```python
from build123d import *

# Parameters (mm, degrees)
SKETCH_R         = 44
SKETCH_R_2       = 30
PAD_DEPTH        = 5
SKETCH001_R      = 44
SKETCH001_R_2    = 41
PAD001_DEPTH     = 65
SKETCH002_R      = 44
SKETCH002_R_2    = 34
PAD002_DEPTH     = 5
HOLE_D           = 3.6
HOLE_DEPTH       = 5
HOLE_CBORE_D     = 6.2
HOLE_CBORE_DEPTH = 3
CHAMFER_SIZE     = 6.9
FILLET_R         = 1
CHAMFER001_SIZE  = 1
CHAMFER002_SIZE  = 3.8
FILLET001_R      = 3
CHAMFER003_SIZE  = 0.2


with BuildPart() as part:
    # Sketch → Pad (new body)
    with BuildSketch(Plane.XY):
        Circle(SKETCH_R)
        Circle(SKETCH_R_2, mode=Mode.SUBTRACT)
    extrude(amount=PAD_DEPTH)

    # Sketch001 (on DatumPlane) → Pad001 (join)
    with BuildSketch(Plane.XY.offset(5)):
        Circle(SKETCH001_R)
        Circle(SKETCH001_R_2, mode=Mode.SUBTRACT)
    extrude(amount=PAD001_DEPTH)

    # Sketch002 (on DatumPlane) → Pad002 (join)
    with BuildSketch(Plane.XY.offset(70)):
        Circle(SKETCH002_R)
        Circle(SKETCH002_R_2, mode=Mode.SUBTRACT)
    extrude(amount=PAD002_DEPTH)

    # Hole
    with Locations(Plane.XY.offset(5)):
        with Locations((-36.6, 0), (18.3, 31.69653), (18.3, -31.69653)):
            CounterBoreHole(HOLE_D / 2, HOLE_CBORE_D / 2, HOLE_CBORE_DEPTH, depth=HOLE_DEPTH)

    # Chamfer
    chamfer_edges = [part.edges().sort_by_distance(p)[0] for p in [
        (-41, 0, 70),
    ]]
    chamfer(chamfer_edges, length=CHAMFER_SIZE)

    # Fillet
    fillet_edges = [part.edges().sort_by_distance(p)[0] for p in [
        (-34, 0, 75),
        (-44, 0, 75),
    ]]
    fillet(fillet_edges, radius=FILLET_R)

    # Chamfer001
    chamfer001_edges = [part.edges().sort_by_distance(p)[0] for p in [
        (-41, 0, 5),
    ]]
    chamfer(chamfer001_edges, length=CHAMFER001_SIZE)

    # Chamfer002
    chamfer002_edges = [part.edges().sort_by_distance(p)[0] for p in [
        (-44, 0, 0),
    ]]
    chamfer(chamfer002_edges, length=CHAMFER002_SIZE)

    # Fillet001
    fillet001_edges = [part.edges().sort_by_distance(p)[0] for p in [
        (-30, 0, 5),
    ]]
    fillet(fillet001_edges, radius=FILLET001_R)

    # Chamfer003
    chamfer003_edges = [part.edges().sort_by_distance(p)[0] for p in [
        (-30, 0, 0),
    ]]
    chamfer(chamfer003_edges, length=CHAMFER003_SIZE)


solid = part.part
```
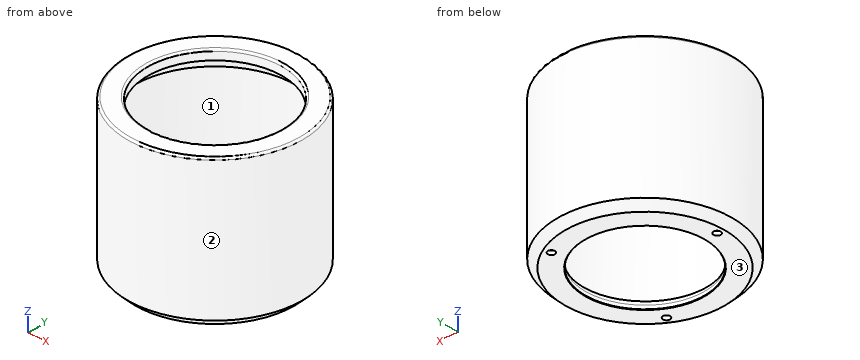
Input: part model. Units: mm. Frame: model coordinates. Face numbers are marked on the shaded views. Give positions to 0.01 mm unless a question says otherwise; leave off trailing zeros. Write each loop counter-clockwise with the first axis right and the second up, starting at its lowest first coordinate (ties: lowest second). Pieces come first, ordered by that corner, then holes. Notation, with made-up numbers: (18, 27) - (61, 27) arc R24 cw to (61, 47) - close; hole circle Ø5 at (12.5, 56). An arc over 180 degrees is marked (long way). Write item = value, one per line. Start each with the question number.
1) Cut plane C-C (y = 0). Give the number of separate pieces and of enclosed holes in the cut face, and give its area (3 significant figures).
2) Pin query (flat end, axial travel): pin 1 (10 mm diameter, centred on x = 21.5, z = 14, fed in from -Y); pin 2 (12 mm diameter, centred on y = 30, z = 10, fed in from -X); pin 3 (1.5 mm diameter, centred on y = 34.5, z = 48, fed in from -X). Return the tip coordinate at first contact, or that it passes through.
3) Draft query along Y for the marked faces 1, 2 and 3. Return one class per face: pulls with the +Y half, pulls with the -Y half, needs draft (parallel to the pull), parting line crosses it, or undercut.
4) Cut plane B-B (z = 60). Return loops of the section in (x, y).
5) Material intervals for L1, parallel to Y at x = 0, z = 72.8; L2, parallel to X at y = -1, z = 62.5; L3, parallel to Y at x = 0, z = 23.5, sorted ascending. Write a range as [from, to].
Answers follow:
q1.separate_pieces = 3
q1.enclosed_holes = 0
q1.area = 634 mm^2
q2.pin_1 = -40.79
q2.pin_2 = -36.88
q2.pin_3 = -28.23
q3.face_1 = undercut
q3.face_2 = parting line crosses it
q3.face_3 = needs draft
q4.outline = circle Ø88 at (0, 0); hole circle Ø82 at (0, 0)
q5.L1 = [-44, -34], [34, 44]
q5.L2 = [-43.99, -40.99], [40.99, 43.99]
q5.L3 = [-44, -41], [41, 44]
